from build123d import *

# Parameters (mm, degrees)
SKETCH1_R           = 12.626048476
SKETCH1_R_2         = 6.35
BOSS_EXTRUDE1_DEPTH = 6.35
BOSS_EXTRUDE2_DEPTH = 6.35
SKETCH4_R           = 3.175
BOSS_EXTRUDE3_DEPTH = 50.8
CUT_EXTRUDE1_START  = -6.35
CUT_EXTRUDE1_DEPTH  = 6.35
SKETCH7_R           = 3.175
BOSS_EXTRUDE4_DEPTH = 57.15
SKETCH7_2_R         = 3.175
CUT_EXTRUDE2_DEPTH  = 25.4
FILLET1_R           = 3.175


with BuildPart() as part:
    # Sketch1 → Boss-Extrude1 (new body)
    with BuildSketch(Plane(origin=(0, 0, 0), x_dir=(0, 0, -1), z_dir=(1, 0, 0))):
        Circle(SKETCH1_R)
        Circle(SKETCH1_R_2, mode=Mode.SUBTRACT)
    extrude(amount=BOSS_EXTRUDE1_DEPTH)

    # Sketch3 → Boss-Extrude2 (add)
    with BuildSketch(Plane(origin=(6.35, 0, 0), x_dir=(0, 0, -1), z_dir=(1, 0, 0))):
        Polygon((-8.994798287, -8.860626609), (-8.994798287, -15.452306957), (10.798615768, -15.452306957), (10.798615768, -6.542705681), (-8.994798287, -6.542705681), align=None)
    extrude(amount=-BOSS_EXTRUDE2_DEPTH)

    # Sketch4 → Boss-Extrude3 (add)
    with BuildSketch(Plane.XZ.offset(15.452306957)):
        with Locations(Location((3.175, 0, 0), (0, 0, 180))):
            Circle(SKETCH4_R)
    extrude(amount=BOSS_EXTRUDE3_DEPTH)

    # Sketch5 → Cut-Extrude1 (cut)
    with BuildSketch(Plane(origin=(6.35, 0, 0), x_dir=(0, 0, -1), z_dir=(1, 0, 0)).offset(CUT_EXTRUDE1_START)):
        with BuildLine():
            Line((-8.994798287, -8.860626609), (-8.994798287, -15.452306957))
            Line((-8.994798287, -15.452306957), (10.798615768, -15.452306957))
            Line((10.798615768, -15.452306957), (10.798615768, -6.542705681))
            ThreePointArc((10.798615768, -6.542705681), (1.46854647, -12.540353719), (-8.994798287, -8.860626609))
        make_face()
    extrude(amount=CUT_EXTRUDE1_DEPTH, mode=Mode.SUBTRACT)


with BuildPart() as cut_extrude1_piece_1:
    # of the separate pieces the step leaves, piece 1, a body of its own (cut_extrude1_pieces)
    add(part.part.solids().sort_by_distance((0, -6.542705681, -10.798615768))[0])



with BuildPart() as cut_extrude1_piece_2:
    # of the separate pieces the step leaves, piece 2, a body of its own (cut_extrude1_pieces)
    add(part.part.solids().sort_by_distance((0, -15.452306957, 0))[0])


with BuildPart() as cut_extrude1_piece_1_1:
    add(cut_extrude1_piece_1.part)

    add(cut_extrude1_piece_2.part)  # Boss-Extrude4 merges Cut-Extrude1 piece 2
    # Sketch7 → Boss-Extrude4 (add)
    with BuildSketch(Plane.XZ.offset(66.252306957)):
        with Locations((3.175, 0)):
            Circle(SKETCH7_R)
    extrude(amount=-BOSS_EXTRUDE4_DEPTH)

    # Sketch7<2> → Cut-Extrude2 (cut)
    with BuildSketch(Plane.XZ.offset(66.252306957)):
        with Locations((3.175, 0)):
            Circle(SKETCH7_2_R)
    extrude(amount=-CUT_EXTRUDE2_DEPTH, mode=Mode.SUBTRACT)

    # Fillet1
    # the kernel refuses this fillet: 3.175 mm, written as the material it takes off along each edge
    with BuildSketch(Plane(origin=(6.35, 0, 0), x_dir=(0, -0.7017735299957855, 0.7124001071008161), z_dir=(0, -0.7124001071008161, -0.7017735299957855))) as fillet1_piece_1:
        with BuildLine():
            CenterArc((12.626048476 - FILLET1_R, FILLET1_R), FILLET1_R, 270, 90)
            Line((12.626048476 - FILLET1_R, 0), (12.626048476, 0))
            Line((12.626048476, 0), (12.626048476, FILLET1_R))
        make_face()
    revolve(axis=Axis((6.35, 0, 0), (-1, 0, 0)), revolution_arc=255.78045899, mode=Mode.SUBTRACT)
    with BuildSketch(Plane(origin=(0, 0, 0), x_dir=(0, -0.5181910787843432, -0.855264874684047), z_dir=(0, -0.855264874684047, 0.5181910787843432))) as fillet1_piece_2:
        with BuildLine():
            CenterArc((12.626048476 - FILLET1_R, FILLET1_R), FILLET1_R, 270, 90)
            Line((12.626048476 - FILLET1_R, 0), (12.626048476, 0))
            Line((12.626048476, 0), (12.626048476, FILLET1_R))
        make_face()
    revolve(axis=Axis((0, 0, 0), (1, 0, 0)), revolution_arc=255.78045899, mode=Mode.SUBTRACT)
    with BuildSketch(Plane(origin=(0, 0, 0), x_dir=(0, -0.5181910787843435, -0.8552648746840469), z_dir=(0, 0.8552648746840469, -0.5181910787843435))) as fillet1_piece_3_section:
        with BuildLine():
            CenterArc((12.626048476 - FILLET1_R, -FILLET1_R), FILLET1_R, 0, 90)
            Line((12.626048476 - FILLET1_R, 0), (12.626048476, 0))
            Line((12.626048476, 0), (12.626048476, -FILLET1_R))
        make_face()
    fillet1_piece_3 = revolve(axis=Axis((0, 0, 0), (-1, 0, 0)), revolution_arc=58.789009325, mode=Mode.PRIVATE)
    fillet1_piece_3 = fillet1_piece_3 - Plane(origin=(3.175, -9.611252213, 0), x_dir=(1, 0, 0), z_dir=(0, -1, 0)) * Cylinder(3.175, 51, mode=Mode.PRIVATE)
    add(fillet1_piece_3, mode=Mode.SUBTRACT)
    with BuildSketch(Plane(origin=(0, 0, 0), x_dir=(0, -1, 0), z_dir=(0, 0, -1))) as fillet1_piece_4_section:
        with BuildLine():
            CenterArc((12.626048476 - FILLET1_R, -FILLET1_R), FILLET1_R, 0, 90)
            Line((12.626048476 - FILLET1_R, 0), (12.626048476, 0))
            Line((12.626048476, 0), (12.626048476, -FILLET1_R))
        make_face()
    fillet1_piece_4 = revolve(axis=Axis((0, 0, 0), (-1, 0, 0)), revolution_arc=45.430531685, mode=Mode.PRIVATE)
    fillet1_piece_4 = fillet1_piece_4 - Plane(origin=(3.175, -10.439695548, 0), x_dir=(1, 0, 0), z_dir=(0, -1, 0)) * Cylinder(3.175, 51, mode=Mode.PRIVATE)
    add(fillet1_piece_4, mode=Mode.SUBTRACT)
    with BuildSketch(Plane(origin=(6.35, 0, 0), x_dir=(0, -1, 0), z_dir=(0, 0, -1))) as fillet1_piece_5_section:
        with BuildLine():
            CenterArc((12.626048476 - FILLET1_R, FILLET1_R), FILLET1_R, 270, 90)
            Line((12.626048476 - FILLET1_R, 0), (12.626048476, 0))
            Line((12.626048476, 0), (12.626048476, FILLET1_R))
        make_face()
    fillet1_piece_5 = revolve(axis=Axis((6.35, 0, 0), (-1, 0, 0)), revolution_arc=45.430531685, mode=Mode.PRIVATE)
    fillet1_piece_5 = fillet1_piece_5 - Plane(origin=(3.175, -10.439696502, 0), x_dir=(1, 0, 0), z_dir=(0, -1, 0)) * Cylinder(3.175, 51, mode=Mode.PRIVATE)
    add(fillet1_piece_5, mode=Mode.SUBTRACT)
    with BuildSketch(Plane(origin=(6.35, 0, 0), x_dir=(0, -0.5181910787843435, -0.8552648746840469), z_dir=(0, 0.8552648746840469, -0.5181910787843435))) as fillet1_piece_6_section:
        with BuildLine():
            CenterArc((12.626048476 - FILLET1_R, FILLET1_R), FILLET1_R, 270, 90)
            Line((12.626048476 - FILLET1_R, 0), (12.626048476, 0))
            Line((12.626048476, 0), (12.626048476, FILLET1_R))
        make_face()
    fillet1_piece_6 = revolve(axis=Axis((6.35, 0, 0), (-1, 0, 0)), revolution_arc=58.789009325, mode=Mode.PRIVATE)
    fillet1_piece_6 = fillet1_piece_6 - Plane(origin=(3.175, -9.611252422, 0), x_dir=(1, 0, 0), z_dir=(0, -1, 0)) * Cylinder(3.175, 51, mode=Mode.PRIVATE)
    add(fillet1_piece_6, mode=Mode.SUBTRACT)


solid = cut_extrude1_piece_1_1.part
Could you check a few things on this model? Use its own coordinates, in mm. Give positions to 0.01 mm unless a question says otherwise; leave off trailing zeros. Write each loop counter-clockwise with the first axis right and the second up, starting at its lowest first coordinate (ties: lowest second). Pieces come first, ordered by that corner, then holes. Notation, with made-up numbers: (-38.5, 8.5) -> (-15.5, 8.5) arc R25 ccw to (-15.5, 21.5) -> close; hole circle Ø6 at (56.25, 15). An arc over 180 degrees is marked (long way). Answer as CSV lines item,"result". Start each with the question number.
(1) If we section it at D-D, the plane x = 5: Write out the boundary of the cut face in (y, z).
(2) If we section it at C-C, the plane y = -16: Write out the boundary of the cut face in (x, z) (3 decimals).
(3) If we section it at B-B, the plane x = 2: Write out the boundary of the cut face in (y, z), and give its area (3 significant figures).
(4) I'm going to push flat-ended pins straight in: pin 1 Ø1 at (x, y) = (1, -22.5) entering from +Z; pin 2 Ø2 at (x, z) = (1, -10) entering from +Y; pin 3 Ø1 at (x, z) = (1, -7.5) entering from +Y. Where does each tip first touch, or does it pass through?
(5) Please list where these lines run through material, in increasing order: line 1 (Y direction, x = 5, z = 0); line 2 (Y direction, x = 5, z = 2.75); line 3 (Z direction, x = 2, y = 3).
(6) If we section it at A-A, the plane y = 0: Write out the boundary of the cut face in (x, z) (3 decimals).
Answer list:
1,outline,"(-40.85, -2.6) -> (-11.77, -2.6) arc R12.05 ccw (long way) to (-11.77, 2.6) -> (-40.85, 2.6) -> close; hole circle Ø12.7 at (0, 0)"
2,outline,"circle Ø6.35 at (3.175, 0)"
3,outline,"(-40.85, -2.95) -> (-12.04, -2.95) arc R12.4 ccw (long way) to (-12.04, 2.95) -> (-40.85, 2.95) -> close; hole circle Ø12.7 at (0, 0)"
3,area,"525 mm^2"
4,pin 1,"z = 2.7"
4,pin 2,"y = 8.02"
4,pin 3,"y = 9.71"
5,line 1,"-40.85 to -6.35, 6.35 to 12.05"
5,line 2,"-11.73 to -5.72, 5.72 to 11.73"
5,line 3,"-12.03 to -5.6, 5.6 to 12.03"
6,outline,"(0, -9.451) arc R3.175 ccw to (6.35, -9.451) -> (6.35, -6.35) -> (0, -6.35) -> close; (0, 6.35) -> (6.35, 6.35) -> (6.35, 9.451) arc R3.175 ccw to (0, 9.451) -> close"
